Check sheet for the modelled part. Datum: model origin and axes. Units: mm. Face numbers are marked on the shaded views. A direction names the side the tool comes from. Give positions to 0.01 mm unless a question says otherwise; leave off trailing zeros. Loops run counter-clockwise (first coordinate to the right, second up) from the corner with the lowest first, then second, coordinate; pieces in that order, holes last. Notation, with made-up numbers: M 71,79 L 81,79 A5 ccw 81,88 Z; hole C 88,43 d11. An arc over 180 degrees is marked long. Put each result on its own line as item: value. Start each with the question number.
```python
from build123d import *

# Parameters (mm, degrees)
SKETCH2_R               = 6.35
BOSS_EXTRUDE1_DEPTH     = 44.45
SKETCH4_W               = 5.08
SKETCH4_H               = 12.7
CUT_EXTRUDE1_DEPTH      = 10.16
SKETCH5_R               = 1.27
CUT_EXTRUDE2_DEPTH      = 9.89
CUT_EXTRUDE2_DEPTH_BACK = 4.81


with BuildPart() as part:
    # Sketch2 → Boss-Extrude1 (new body)
    with BuildSketch(Plane.XY):
        Circle(SKETCH2_R)
    extrude(amount=BOSS_EXTRUDE1_DEPTH)

    # Sketch3 → Revolve1 (revolve)
    with BuildSketch(Plane(origin=(0, 0, 0), x_dir=(0, 0, -1), z_dir=(1, 0, 0))):
        Polygon((-50.8, 0), (-44.45, 6.35), (-44.45, 0), align=None)
    revolve(axis=Axis((0, 0, 50.8), (0, 0, -1)))

    # Sketch4 → Cut-Extrude1 (cut)
    with BuildSketch(Plane(origin=(0, 0, 0), x_dir=(-1, 0, 0), z_dir=(0, 0, -1))):
        Rectangle(SKETCH4_W, SKETCH4_H)
    extrude(amount=-CUT_EXTRUDE1_DEPTH, mode=Mode.SUBTRACT)

    # Sketch5 → Cut-Extrude2 (cut, two sides)
    with BuildSketch(Plane.ZY.offset(-2.54)) as cut_extrude2_sk:
        with Locations((3.81, 0)):
            Circle(SKETCH5_R)
    extrude(amount=CUT_EXTRUDE2_DEPTH, mode=Mode.SUBTRACT)
    extrude(cut_extrude2_sk.sketch, amount=-CUT_EXTRUDE2_DEPTH_BACK, mode=Mode.SUBTRACT)


solid = part.part
```
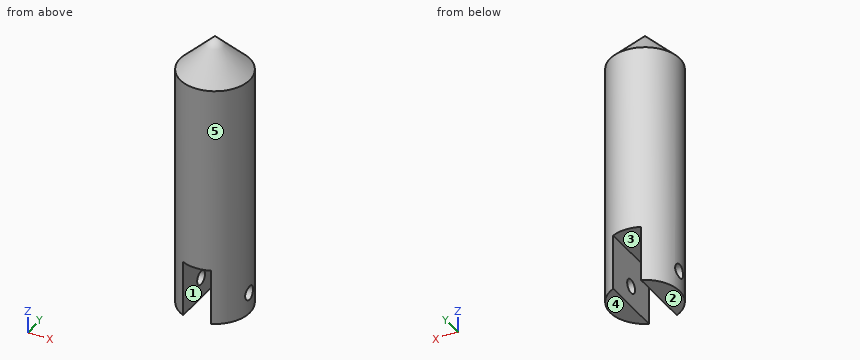
Q1. Section check B-B, the plane z = 17.5. Record the cut outline in (x, y), then the cut area to 3 significant figures.
Q2. Mould release check, pull along X, two halves, no side actions. Record for the marked faces 3, 4 and 5: pulls with the +X half, pulls with the -X half, needs draft (parallel to the pull), parting line crosses it, or undercut.
Q3. Access from +Z, -Z, +X, -X, +Y, -Y to the whole of each face (thin tool, end or side, straight path). Record for the marked faces 1 and 2.
Q4. Section check A-A, the plane z = 3.81. Record the cut outline in (x, y).
Q5. Depth check by flat-ended pin: P1, Ø6, axis at y = 3.5, z = 42.5, coming from the +X side; P2, Ø3, axis at y = -3, z = 21, coming from the -X side; P3, Ø1, axis at x = -1, z = 18, coming from the -Y side. Enter the tip coordinate at first touch or a pass-through.
Q6. Thickness scan on line 1 along Y through (x, z) = (4.1, 3.81); line 2 along X through (y, z) = (0.25, 16); line 3 along Z through (x, y) = (-4.8, 0). Record the ranges inside material, lowest first. Write a range as [from, to].
Found:
1. outline: C 0,0 d12.7
1. area: 127 mm^2
2. face 3: undercut
2. face 4: needs draft
2. face 5: parting line crosses it
3. face 1: -Z, +Y, -Y
3. face 2: -Z, +X, -X, +Y, -Y
4. outline: M -6.22,-1.27 A6.35 ccw -2.54,-5.82 L -2.54,-1.27 Z; M -6.22,1.27 L -2.54,1.27 L -2.54,5.82 A6.35 ccw Z; M 2.54,-5.82 A6.35 ccw 6.22,-1.27 L 2.54,-1.27 Z; M 2.54,1.27 L 6.22,1.27 A6.35 ccw 2.54,5.82 Z
5. P1: stops at x = 6.33
5. P2: stops at x = -6.17
5. P3: stops at y = -6.33
6. line 1: y = [-4.85, -1.27], [1.27, 4.85]
6. line 2: x = [-6.35, 6.35]
6. line 3: z = [0, 2.54], [5.08, 46]
